Job drawing, mm, ordinate dimensions from the low corner. One solid piece. A direction names the side the tool comes from. Coordinates: 2 decimals unless noted, no trailing zeros. Order: outer loops, then holes, each group sorted by start corner. A loop starts at its lowest first (then second) coordinate and runs counter-clockwise, first axis right, second up. Notation, with made-up numbers: (28, 12.25) - (73, 12.25) arc R19 cw to (73, 30.25) - close; hole circle Ø8 at (88, 72). An arc over 180 degrees is marked (long way). Use a Markdown table: item, result. Add a question column.
1) Drop flat-ended pins along their axis: P1, Ø2, axis at x = 1, z = 2, coming from the +Y side; P2, Ø2, axis at x = 4, y = 2.5, coming from the -Z side; P3, Ø0.9, axis at y = 5.5, z = 5.5, coming from the +X side; P4, Ø0.6, axis at y = 7.5, z = 1, coming from the -X side. Give the stop position or say it passes through.
2) Tool access for the marked faces 1 and 2: list every direction of +Z, -Z, +X, -X, +Y, -Y with a clear straight run to the whole face (end or side of a thin tool).
3) Wall check: L1, parallel to Y at x = 3, z = 5.75; L2, parallel to Y at x = 3.25, z = 4; L3, parallel to X at y = 8.5, z = 5.75. Give the ranges that are in metal, low to high. Write a range as [from, to].
4) Saw through at D-D on x = 0.5. List the corners of the cut face in (y, z), then the cut area to 3 significant figures.
5) Saw through at A-A on y = 11. List the corners of the cut face in (x, z).
6) Saw through at B-B on z = 5.5. List the corners of the cut face in (x, y), then the cut area to 3 significant figures.
7) Saw through at C-C on x = 4. List the corners of the cut face in (y, z).
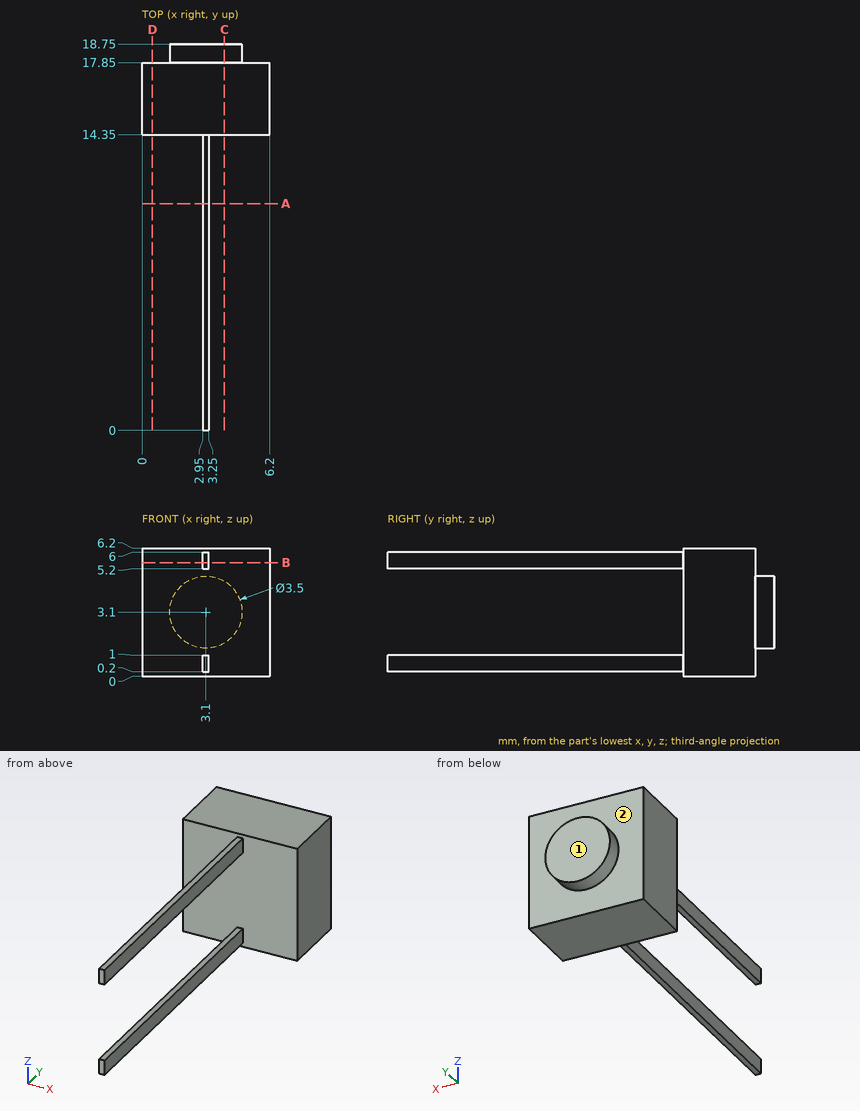
Results are:
| question | item | result |
|---|---|---|
| 1 | P1 | y = 18.75 |
| 1 | P2 | z = 0.2 |
| 1 | P3 | x = 3.25 |
| 1 | P4 | x = 2.95 |
| 2 | face 1 | +Z, -Z, +X, -X, +Y |
| 2 | face 2 | +Y |
| 3 | L1 | [0, 17.85] |
| 3 | L2 | [14.35, 18.75] |
| 3 | L3 | [2.95, 3.25] |
| 4 | outline | (14.35, 0) - (17.85, 0) - (17.85, 6.2) - (14.35, 6.2) - close |
| 4 | area | 21.7 mm2 |
| 5 | outline | (2.95, 0.2) - (3.25, 0.2) - (3.25, 1) - (2.95, 1) - close; (2.95, 5.2) - (3.25, 5.2) - (3.25, 6) - (2.95, 6) - close |
| 6 | outline | (0, 14.35) - (2.95, 14.35) - (2.95, 0) - (3.25, 0) - (3.25, 14.35) - (6.2, 14.35) - (6.2, 17.85) - (0, 17.85) - close |
| 6 | area | 26.0 mm2 |
| 7 | outline | (14.35, 0) - (17.85, 0) - (17.85, 1.6) - (18.75, 1.6) - (18.75, 4.6) - (17.85, 4.6) - (17.85, 6.2) - (14.35, 6.2) - close |
